from build123d import *

# Parameters (mm, degrees)
F0_R     = 3.175
F1_DEPTH = 13.49375
F2_R     = 25.4
F4_W     = 266.7
F4_H     = 238.125
F5_DEPTH = 13.49375
F3_R     = 2.38125
F6_DEPTH = 13.49475
F7_R     = 50.8
F8_R     = 12.7


with BuildPart() as f1:
    # F0 (on Top) → F1 (new body)
    with BuildSketch(Plane.XY):
        with BuildLine():
            Line((133.35, -146.05), (133.35, 146.05))
            Line((133.35, 146.05), (-133.35, 146.05))
            Line((-133.35, 146.05), (-133.35, 63.5))
            ThreePointArc((-133.35, 63.5), (-69.85, 0), (-133.35, -63.5))
            Line((-133.35, -63.5), (-133.35, -146.05))
            Line((-133.35, -146.05), (133.35, -146.05))
        make_face()
        with Locations((0, -88.9)):
            Circle(F0_R, mode=Mode.SUBTRACT)
        with Locations((-44.45, 88.9)):
            Circle(F0_R, mode=Mode.SUBTRACT)
        with Locations((82.55, 88.9)):
            Circle(F0_R, mode=Mode.SUBTRACT)
    extrude(amount=F1_DEPTH)

    # F2
    f2_edges = [f1.edges().sort_by_distance(p)[0] for p in [
        (-133.35, -63.5, 6.746875),
        (-133.35, 63.5, 6.746875),
    ]]
    fillet(f2_edges, radius=F2_R)

    # F4 (on face) → F5 (join, through all)
    with BuildSketch(Plane.XY.offset(13.49375)):
        with Locations((0, 265.1125)):
            Rectangle(F4_W, F4_H)
    extrude(amount=-F5_DEPTH)

    # F3 (on face) → F6 (cut, through all)
    with BuildSketch(Plane.XY.offset(13.49375)):
        with Locations((-107.95, -139.7)):
            Circle(F3_R)
        with Locations((-6.35, -139.7)):
            Circle(F3_R)
        with Locations((-6.35, 159.54375)):
            Circle(F3_R)
        with Locations((-107.95, 159.54375)):
            Circle(F3_R)
    extrude(amount=-F6_DEPTH, mode=Mode.SUBTRACT)

    # F7
    f7_edges = [f1.edges().sort_by_distance(p)[0] for p in [
        (133.35, -146.05, 6.746875),
        (133.35, 384.175, 6.746875),
        (-133.35, 384.175, 6.746875),
    ]]
    fillet(f7_edges, radius=F7_R)

    # F8
    f8_edges = [f1.edges().sort_by_distance(p)[0] for p in [
        (-133.35, -146.05, 6.746875),
    ]]
    fillet(f8_edges, radius=F8_R)


solid = f1.part
Read the model definition and answer for the solid it produces. Units are mm, in the model's axes. A direction names the side the tool comes from. Give positions to 0.01 mm unless a question says otherwise; leave off trailing zeros. Loops run counter-clockwise (first coordinate to the right, second up) from the corner with the lowest first, then second, coordinate; pieces in that order, holes last. Notation, with made-up numbers: (45, 53.25) - (74, 53.25) arc R20 ccw to (74, 70.25) - close; hole circle Ø8 at (87, -11). An arc over 180 degrees is marked (long way). Answer as CSV lines item,"result". Start each with the question number.
1) Which of the six approach directions +Z, -Z, +X, -X, +Y, -Y give full straight-line access (tool end or side, diameter ignored) to faces 1 (the face through (118.864, -130.774, 6.841)), 2 (the face through (-128.45, 70.2, 6.84))?
2) Determine the mould class of faces 3 (the face through (-2, 123, 13.494)), 4 (the face through (-128.45, -70.2, 6.84)), 5 (the face through (-1, 384.175, 7)) for opening direction Y: released by +Y, released by -Y, zero draft, split by the parting line, or undercut.
3) Straight lines are drawn through the part: L1, parallel to X at y = -139.7, z = 2.5; L2, parallel to Y at x = -44, z = 6.25 (3 decimals); L3, parallel to Y at x = -96.5, z = 7.5. For each, find the intervals that lie inside material, in ascending order. Write a range as from..to.
4) Each of these flat-tipped pins is pushed along its axis until it touches: pin 1 Ø8 at (y, z) = (-24.5, 9.5) entering from -X; pin 2 Ø2 at (y, z) = (-4, 9.5) entering from -X. Where does it stop, or does it pass through?
5) Find section A-A (z = 5). State how many separate pieces and enclosed holes the cut face has, then the cut area to 3 significant figures.
6) Find section B-B (x = -88.5). Write down the section's boundary in (y, z).
Findings below:
1,face 1,"+Z, -Z, +X, -Y"
1,face 2,"+Z, -Z, -X"
2,face 3,"zero draft"
2,face 4,"undercut"
2,face 5,"released by +Y"
3,L1,"-131.65..-110.33, -105.57..-8.73, -3.97..107.14"
3,L2,"-146.05..85.757, 92.043..384.175"
3,L3,"-146.05..-51.71, 51.71..382.22"
4,pin 1,"x = -76.6"
4,pin 2,"x = -70.05"
5,separate pieces,"1"
5,enclosed holes,"7"
5,area,"133,000 mm^2"
6,outline,"(-146.05, 0) - (-44.95, 0) - (-44.95, 13.49) - (-146.05, 13.49) - close; (44.95, 0) - (383.83, 0) - (383.83, 13.49) - (44.95, 13.49) - close"
